from build123d import *

# Parameters (mm, degrees)
SKETCH_1_R           = 4
EXTRUDE_1_DEPTH      = 17.8
SKETCH_2_R           = 1.8
EXTRUDE_2_DEPTH      = 2.5
SKETCH_3_R           = 1.8
EXTRUDE_3_DEPTH      = 2.5
SKETCH_4_R           = 4
EXTRUDE_4_DEPTH      = 6.45
EXTRUDE_4_DEPTH_BACK = 6.45
SKETCH_5_R           = 1.8
EXTRUDE_5_DEPTH      = 2
SKETCH_6_R           = 1.8
EXTRUDE_6_DEPTH      = 2


with BuildPart() as part:
    # Sketch 1 → Extrude 1 (new body)
    with BuildSketch(Plane.XY):
        Circle(SKETCH_1_R)
    extrude(amount=EXTRUDE_1_DEPTH)

    # Sketch 2 → Extrude 2 (add)
    with BuildSketch(Plane.XY.offset(17.8)):
        Circle(SKETCH_2_R)
    extrude(amount=EXTRUDE_2_DEPTH)

    # Sketch 3 → Extrude 3 (add)
    with BuildSketch(Plane(origin=(0, 0, 0), x_dir=(-1, 0, 0), z_dir=(0, 0, -1))):
        Circle(SKETCH_3_R)
    extrude(amount=EXTRUDE_3_DEPTH)

    # Sketch 4 → Extrude 4 (add, two sides)
    with BuildSketch(Plane(origin=(0, 0, 0), x_dir=(1, 0, 0), z_dir=(0, 1, 0))) as extrude_4_sk:
        with Locations((0, -8.9)):
            Circle(SKETCH_4_R)
    extrude(amount=EXTRUDE_4_DEPTH)
    extrude(extrude_4_sk.sketch, amount=-EXTRUDE_4_DEPTH_BACK)

    # Sketch 5 → Extrude 5 (add)
    with BuildSketch(Plane(origin=(0, -6.45, 0), x_dir=(-1, 0, 0), z_dir=(0, -1, 0))):
        with Locations((0, -8.9)):
            Circle(SKETCH_5_R)
    extrude(amount=EXTRUDE_5_DEPTH)

    # Sketch 6 → Extrude 6 (add)
    with BuildSketch(Plane(origin=(0, 6.45, 0), x_dir=(1, 0, 0), z_dir=(0, 1, 0))):
        with Locations((0, -8.9)):
            Circle(SKETCH_6_R)
    extrude(amount=EXTRUDE_6_DEPTH)


solid = part.part
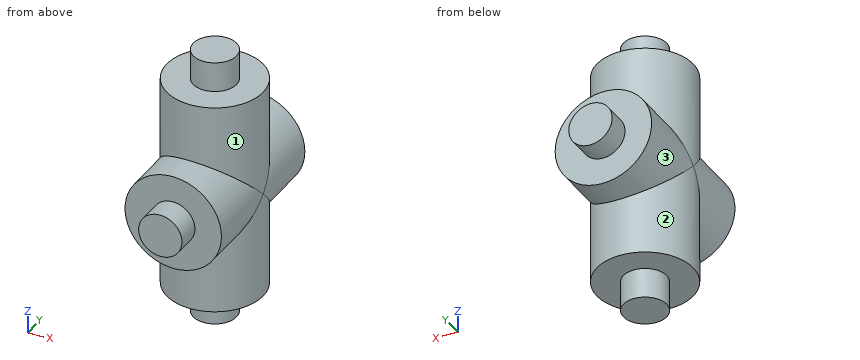
The model under review builds one solid part; all positions refer to its coordinate system, in mm. Face numbers are marked on the shaded views. A direction names the side the tool comes from. Give positions to 0.01 mm unless a question says otherwise; leave off trailing zeros. Loops run counter-clockwise (first coordinate to the right, second up) from the corner with the lowest first, then second, coordinate; pieces in that order, holes last. Notation, with made-up numbers: (-22.75, 66) -> (-7.75, 66) arc R18 ccw to (-7.75, 77) -> close; hole circle Ø9 at (52.5, -3.75). An arc over 180 degrees is marked (long way). Put each result on its own line as item: value. Start each with the question number.
1. Clearance check with flat-ended pins moving along their axes: P1, Ø3, axis at x = -1.5, z = 12, coming from the +Y side; P2, Ø4, axis at y = 3.5, z = 1, coming from the +X side; P3, Ø2, axis at y = 6.5, z = 5.5, coming from the -X side. State where each tip first meets the part, or that it passes through.
2. We need section D-D on x = -1.25. State the section outline as (y, z) points.
3. We need section B-B on z = 8. State the section outline as (x, y) points, then the cut area to 3 significant figures.
4. Wall thickness on probe 1 along Z at (x, y) = (-3, -1); probe 2 along Y at (x, z) = (-3, 15.5); probe 3 along Z at (x, y) = (0.75, -5.5): over which ranges is each line inside the solid? List them lowest first.
5. We need section C-C on y = 7. State the section outline as (x, z) points, then the cut area to 3 significant figures.
6. For the marked faces 1, 2 and 3, list the 3-axis set-ups (+Z, -Z, +X, -X, +Y, -Y) from which the entire face can be reached by the end or side of a thin tool; tool diameter is ignored.
7. We need section A-A on x = 0. State the section outline as (y, z) points.
Determined:
1. P1: y = 6.45
1. P2: x = 3.71
1. P3: x = -3.2
2. outline: (-8.45, 7.6) -> (-6.45, 7.6) -> (-6.45, 5.1) -> (-3.8, 5.1) -> (-3.8, 0) -> (-1.3, 0) -> (-1.3, -2.5) -> (1.3, -2.5) -> (1.3, 0) -> (3.8, 0) -> (3.8, 5.1) -> (6.45, 5.1) -> (6.45, 7.6) -> (8.45, 7.6) -> (8.45, 10.2) -> (6.45, 10.2) -> (6.45, 12.7) -> (3.8, 12.7) -> (3.8, 17.8) -> (1.3, 17.8) -> (1.3, 20.3) -> (-1.3, 20.3) -> (-1.3, 17.8) -> (-3.8, 17.8) -> (-3.8, 12.7) -> (-6.45, 12.7) -> (-6.45, 10.2) -> (-8.45, 10.2) -> close
3. outline: (-3.9, -6.45) -> (-1.56, -6.45) -> (-1.56, -8.45) -> (1.56, -8.45) -> (1.56, -6.45) -> (3.9, -6.45) -> (3.9, -0.9) arc R4 ccw to (3.9, 0.9) -> (3.9, 6.45) -> (1.56, 6.45) -> (1.56, 8.45) -> (-1.56, 8.45) -> (-1.56, 6.45) -> (-3.9, 6.45) -> (-3.9, 0.9) arc R4 ccw to (-3.9, -0.9) -> close
3. area: 113 mm^2
4. probe 1: 0 to 17.8
4. probe 2: -2.65 to 2.65
4. probe 3: 4.97 to 12.83
5. outline: circle Ø3.6 at (0, 8.9)
5. area: 10.2 mm^2
6. face 1: +Z
6. face 2: -Z
6. face 3: +Y
7. outline: (-8.45, 7.1) -> (-6.45, 7.1) -> (-6.45, 4.9) -> (-4, 4.9) -> (-4, 0) -> (-1.8, 0) -> (-1.8, -2.5) -> (1.8, -2.5) -> (1.8, 0) -> (4, 0) -> (4, 4.9) -> (6.45, 4.9) -> (6.45, 7.1) -> (8.45, 7.1) -> (8.45, 10.7) -> (6.45, 10.7) -> (6.45, 12.9) -> (4, 12.9) -> (4, 17.8) -> (1.8, 17.8) -> (1.8, 20.3) -> (-1.8, 20.3) -> (-1.8, 17.8) -> (-4, 17.8) -> (-4, 12.9) -> (-6.45, 12.9) -> (-6.45, 10.7) -> (-8.45, 10.7) -> close
